For this review, take the finished solid that the model builds, in its own axes (mm). Give positions to 0.01 mm unless a question says otherwise; leave off trailing zeros. Write each loop counter-clockwise with the first axis right and the second up, starting at its lowest first coordinate (ties: lowest second). Pieces come first, ordered by that corner, then holes. Notation, with made-up numbers: M 57.25,74.25 L 103.25,74.25 A19 ccw 103.25,102.25 Z; hole C 80.5,34.5 d1. An arc over 180 degrees is marked long. Write item = value, one per line.
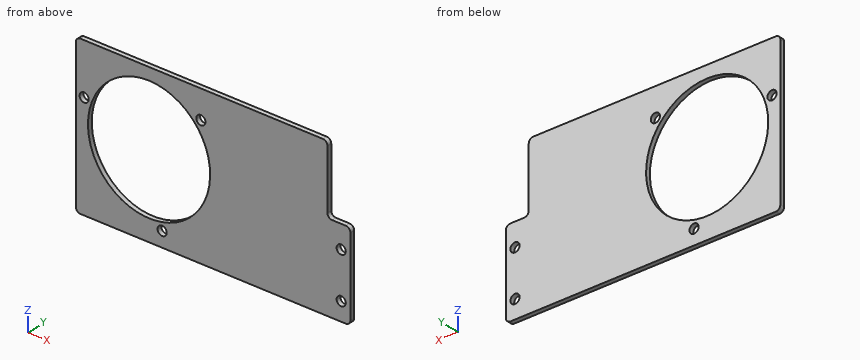
```python
from build123d import *

# Parameters (mm, degrees)
SKETCH1_R           = 84.7725
SKETCH1_R_2         = 6.35
BOSS_EXTRUDE1_DEPTH = 6.35


with BuildPart() as part:
    # Sketch1 → Boss-Extrude1 (new body)
    with BuildSketch(Plane(origin=(0, 0, 0), x_dir=(1, 0, 0), z_dir=(0, 1, 0))):
        with BuildLine():
            Line((273.05, 114.3), (-95.25, 114.3))
            ThreePointArc((-95.25, 114.3), (-99.740128061, 112.440128061), (-101.6, 107.95))
            Line((-101.6, 107.95), (-101.6, -95.25))
            ThreePointArc((-101.6, -95.25), (-99.740128061, -99.740128061), (-95.25, -101.6))
            Line((-95.25, -101.6), (241.3, -101.6))
            ThreePointArc((241.3, -101.6), (245.790128061, -99.740128061), (247.65, -95.25))
            Line((247.65, -95.25), (247.65, -12.7))
            ThreePointArc((247.65, -12.7), (249.509871939, -8.209871939), (254, -6.35))
            Line((254, -6.35), (273.05, -6.35))
            ThreePointArc((273.05, -6.35), (277.540128061, -4.490128061), (279.4, 0))
            Line((279.4, 0), (279.4, 107.95))
            ThreePointArc((279.4, 107.95), (277.540128061, 112.440128061), (273.05, 114.3))
        make_face()
        with Locations(Location((0, 0, 0), (0, 0, 270))):
            Circle(SKETCH1_R, mode=Mode.SUBTRACT)
        with Locations(Location((-90.060644326, -31.010366712, 0), (0, 0, 270))):
            Circle(SKETCH1_R_2, mode=Mode.SUBTRACT)
        with Locations(Location((18.17455681, 93.499989223, 0), (0, 0, 270))):
            Circle(SKETCH1_R_2, mode=Mode.SUBTRACT)
        with Locations(Location((71.886087516, -62.489622511, 0), (0, 0, 270))):
            Circle(SKETCH1_R_2, mode=Mode.SUBTRACT)
        with Locations(Location((266.7, 88.9, 0), (0, 0, 270))):
            Circle(SKETCH1_R_2, mode=Mode.SUBTRACT)
        with Locations(Location((266.7, 25.4, 0), (0, 0, 270))):
            Circle(SKETCH1_R_2, mode=Mode.SUBTRACT)
    extrude(amount=BOSS_EXTRUDE1_DEPTH)


solid = part.part
```
1. Insertion check: P1, Ø11.5, axis at x = 266.7, z = -25.4, coming from the +Y side; P2, Ø1.9, axis at x = 266, y = 4.5, coming from the +Z side; P3, Ø3, axis at y = 2, z = 62.5, coming from the +X side. Each pin has a flat end and moves straight along its axis. Give the tip position at first contact, or say it passes through.
Responses:
P1 = through
P2 = 6.35
P3 = 247.65
2. For line 1 along Z through (x, y) = (266.7, 2.5); line 2 along Z through (x, y) = (1, 2.25); line 3 along X through (y, z) = (4.25, -25.4), list the stretches that pass through material, from the lowest coordinate up. Write a range as from..to.
Responses:
line_1 = -114.3..-95.25, -82.55..-31.75, -19.05..6.35
line_2 = -114.3..-84.77, 84.77..101.6
line_3 = -101.6..-80.88, 80.88..260.35, 273.05..279.4
3. We need section B-B, the plane z = 43.5. Write out the cut boundary in (x, y).
Responses:
outline = M -101.6,0 L -72.76,0 L -72.76,6.35 L -101.6,6.35 Z; M 72.76,0 L 247.65,0 L 247.65,6.35 L 72.76,6.35 Z
4. We need section D-D, the plane z = -25.4. Write out the cut boundary in (x, y), then the cut area to 3 significant figures.
Responses:
outline = M -101.6,0 L -80.88,0 L -80.88,6.35 L -101.6,6.35 Z; M 80.88,0 L 260.35,0 L 260.35,6.35 L 80.88,6.35 Z; M 273.05,0 L 279.4,0 L 279.4,6.35 L 273.05,6.35 Z
area = 1,310 mm2
5. We need section C-C, the plane x = 0. Write out the cut boundary in (y, z).
Responses:
outline = M 0,-114.3 L 6.35,-114.3 L 6.35,-84.77 L 0,-84.77 Z; M 0,84.77 L 6.35,84.77 L 6.35,101.6 L 0,101.6 Z
6. We need section A-A, the plane x = 266.7. Write out the cut boundary in (y, z), then the cut area to 3 significant figures.
Responses:
outline = M 0,-114.3 L 6.35,-114.3 L 6.35,-95.25 L 0,-95.25 Z; M 0,-82.55 L 6.35,-82.55 L 6.35,-31.75 L 0,-31.75 Z; M 0,-19.05 L 6.35,-19.05 L 6.35,6.35 L 0,6.35 Z
area = 605 mm2
